Here's how the part is built. I have some questions about the finished solid (model axes, mm). Face numbers are marked on the shaded views. A direction names the side the tool comes from. Round coordinates to 2 decimals unless told otherwise and drop trailing zeros. Order: outer loops, then holes, each group sorted by start corner. A loop starts at its lowest first (then second) coordinate and runs counter-clockwise, first axis right, second up. Notation, with made-up numbers: (28.25, 12.5) -> (71.25, 12.5) arc R35 cw to (71.25, 49.5) -> close; hole circle Ø3 at (86, -37.75). An arc over 180 degrees is marked (long way). One line per item, written item: value.
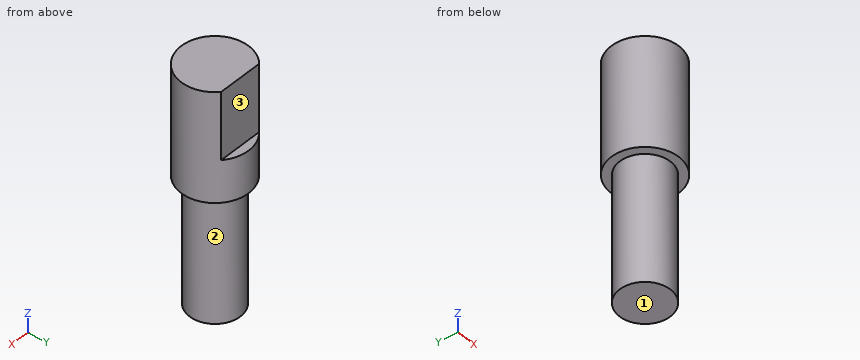
```python
from build123d import *

# Parameters (mm, degrees)
SKETCH_1_R          = 4
EXTRUDE_1_DEPTH     = 28
SKETCH_2_W          = 11.268608601
SKETCH_2_H          = 1.937161227
CUT_EXTRUDE_1_DEPTH = 15
SKETCH_3_W          = 8.764473356
SKETCH_3_H          = 2.433263492
CUT_EXTRUDE_2_DEPTH = 8
SKETCH_4_R          = 4.002706421
CUT_EXTRUDE_3_DEPTH = 15
SKETCH_5_R          = 3
EXTRUDE_2_DEPTH     = 15


with BuildPart() as part:
    # 스케치1 → 보스-돌출1 (new body)
    with BuildSketch(Plane.XY):
        Circle(SKETCH_1_R)
    extrude(amount=EXTRUDE_1_DEPTH)

    # 스케치2 → 컷-돌출1 (cut)
    with BuildSketch(Plane(origin=(0, 0, 0), x_dir=(-1, 0, 0), z_dir=(0, 0, -1))):
        with Locations((0.295298967, 3.968580614)):
            Rectangle(SKETCH_2_W, SKETCH_2_H)
    extrude(amount=-CUT_EXTRUDE_1_DEPTH, mode=Mode.SUBTRACT)

    # 스케치3 → 컷-돌출2 (cut)
    with BuildSketch(Plane.XY.offset(28)):
        with Locations((0.244916085, 4.216631746)):
            Rectangle(SKETCH_3_W, SKETCH_3_H)
    extrude(amount=-CUT_EXTRUDE_2_DEPTH, mode=Mode.SUBTRACT)

    # 스케치4 → 컷-돌출3 (cut)
    with BuildSketch(Plane(origin=(0, 0, 0), x_dir=(-1, 0, 0), z_dir=(0, 0, -1))):
        Circle(SKETCH_4_R)
    extrude(amount=-CUT_EXTRUDE_3_DEPTH, mode=Mode.SUBTRACT)

    # 스케치5 → 보스-돌출2 (add)
    with BuildSketch(Plane(origin=(0, 0, 15), x_dir=(-1, 0, 0), z_dir=(0, 0, -1))):
        Circle(SKETCH_5_R)
    extrude(amount=EXTRUDE_2_DEPTH)


solid = part.part
```
Q1. I want a section at A-A on x = 0. Write out the boundary of the cut face in (y, z), then the cut area to 3 significant figures.
Answers:
outline: (-4, 15) -> (-3, 15) -> (-3, 0) -> (3, 0) -> (3, 15) -> (4, 15) -> (4, 20) -> (3, 20) -> (3, 28) -> (-4, 28) -> close
area: 186 mm2
Q2. I need wall thicknesses on line 1 along Z through (x, y) = (0.75, 3.5); line 2 along Z through (x, y) = (2.25, -2.75); line 3 along Y through (x, z) = (-3, 16). Which ranges of each line are inside material? Lowest first, please.
Answers:
line 1: 15 to 20
line 2: 15 to 28
line 3: -2.65 to 2.65
Q3. I want a section at D-D on z = 19. Write out the boundary of the cut face in (x, y), then the cut area to 3 significant figures.
Answers:
outline: circle Ø8 at (0, 0)
area: 50.3 mm2
Q4. For P1, Ø2, axis at y = 0.5, z = 7, coming from the +X side; P2, Ø1.6, axis at x = -1, z = 25, coming from the +Y side; P3, Ø2, axis at x = -2, z = 18, coming from the +Y side, each with a flat end and sliding along its axis, tell me the tip position at first contact or that it passes through.
Answers:
P1: x = 3
P2: y = 3
P3: y = 3.87
Q5. I want a section at C-C on z = 23. Write out the boundary of the cut face in (x, y).
Answers:
outline: (-2.65, 3) arc R4 ccw (long way) to (2.65, 3) -> close
Q6. I want a section at B-B on y = 0. Write out the boundary of the cut face in (x, z).
Answers:
outline: (-4, 15) -> (-3, 15) -> (-3, 0) -> (3, 0) -> (3, 15) -> (4, 15) -> (4, 28) -> (-4, 28) -> close
Q7. Which directions (+Z, -Z, +X, -X, +Y, -Y) give clear straight access to the entire face, cutting with the end or side of a thin tool? Please do the marked faces 1, 2 and 3.
Answers:
face 1: -Z, +X, -X, +Y, -Y
face 2: -Z
face 3: +Z, +X, -X, +Y
